from build123d import *

# Parameters (mm, degrees)
SKETCH021_W   = 231.14
SKETCH021_H   = 231.14
SKETCH021_R   = 1.5875
SKETCH021_W_2 = 7.62
SKETCH021_H_2 = 7.62
PAD003_DEPTH  = 6.35
FILLET_R      = 1.27
FILLET001_R   = 1.27
SKETCH025_W   = 9
SKETCH025_H   = 18
POCKET_DEPTH  = 6.35
FILLET002_R   = 2


with BuildPart() as part:
    # Sketch021 → Pad003 (new body)
    with BuildSketch(Plane.XY):
        with Locations((0, -18.161)):
            Rectangle(SKETCH021_W, SKETCH021_H)
        with Locations((-111.76, -129.921)):
            Circle(SKETCH021_R, mode=Mode.SUBTRACT)
        with Locations((111.76, -129.921)):
            Circle(SKETCH021_R, mode=Mode.SUBTRACT)
        with Locations((111.76, 93.599)):
            Circle(SKETCH021_R, mode=Mode.SUBTRACT)
        with Locations((-111.76, 93.599)):
            Circle(SKETCH021_R, mode=Mode.SUBTRACT)
        with Locations((-76.2, 58.42)):
            Circle(SKETCH021_R, mode=Mode.SUBTRACT)
        with Locations((76.2, 58.42)):
            Circle(SKETCH021_R, mode=Mode.SUBTRACT)
        with Locations((76.2, -93.98)):
            Circle(SKETCH021_R, mode=Mode.SUBTRACT)
        with Locations((-76.2, -93.98)):
            Circle(SKETCH021_R, mode=Mode.SUBTRACT)
        with BuildLine():
            Line((-86.995, 74.968261), (-86.995, 78.994))
            ThreePointArc((-86.995, 78.994), (-90.17, 82.169), (-93.345, 78.994))
            Line((-93.345, 78.994), (-93.345, 74.968261))
            ThreePointArc((-93.345, 74.968261), (-90.17, 63.119), (-86.995, 74.968261))
        make_face(mode=Mode.SUBTRACT)
        with Locations((7.62, 86.36)):
            Rectangle(SKETCH021_W_2, SKETCH021_H_2, mode=Mode.SUBTRACT)
        with Locations((-22.86, 86.36)):
            Rectangle(SKETCH021_W_2, SKETCH021_H_2, mode=Mode.SUBTRACT)
        with Locations((-38.1, 86.36)):
            Rectangle(SKETCH021_W_2, SKETCH021_H_2, mode=Mode.SUBTRACT)
        with Locations((-7.62, 86.36)):
            Rectangle(SKETCH021_W_2, SKETCH021_H_2, mode=Mode.SUBTRACT)
        with Locations((-68.58, 86.36)):
            Rectangle(SKETCH021_W_2, SKETCH021_H_2, mode=Mode.SUBTRACT)
        with Locations((-53.34, 86.36)):
            Rectangle(SKETCH021_W_2, SKETCH021_H_2, mode=Mode.SUBTRACT)
        with BuildLine():
            Line((86.995, 78.994), (86.995, 74.968261))
            ThreePointArc((86.995, 74.968261), (90.17, 63.119), (93.345, 74.968261))
            Line((93.345, 78.994), (93.345, 74.968261))
            ThreePointArc((93.345, 78.994), (90.17, 82.169), (86.995, 78.994))
        make_face(mode=Mode.SUBTRACT)
        with BuildLine():
            Line((-86.995, -111.290261), (-86.995, -115.316))
            ThreePointArc((-93.345, -115.316), (-90.17, -118.491), (-86.995, -115.316))
            Line((-93.345, -115.316), (-93.345, -111.290261))
            ThreePointArc((-86.995, -111.290261), (-90.17, -99.441), (-93.345, -111.290261))
        make_face(mode=Mode.SUBTRACT)
        with BuildLine():
            Line((93.345, -111.290261), (93.345, -115.316))
            ThreePointArc((86.995, -115.316), (90.17, -118.491), (93.345, -115.316))
            Line((86.995, -115.316), (86.995, -111.290261))
            ThreePointArc((93.345, -111.290261), (90.17, -99.441), (86.995, -111.290261))
        make_face(mode=Mode.SUBTRACT)
    extrude(amount=-PAD003_DEPTH)

    # Fillet
    fillet_edges = [part.edges().sort_by_distance(p)[0] for p in [
        (-72.39, 90.17, -3.175),
        (-64.77, 90.17, -3.175),
        (-64.77, 82.55, -3.175),
        (-72.39, 82.55, -3.175),
        (-57.15, 90.17, -3.175),
        (-49.53, 90.17, -3.175),
        (-49.53, 82.55, -3.175),
        (-57.15, 82.55, -3.175),
        (-41.91, 90.17, -3.175),
        (-34.29, 90.17, -3.175),
        (-34.29, 82.55, -3.175),
        (-41.91, 82.55, -3.175),
        (-26.67, 90.17, -3.175),
        (-19.05, 90.17, -3.175),
        (-19.05, 82.55, -3.175),
        (-26.67, 82.55, -3.175),
        (-11.43, 90.17, -3.175),
        (-3.81, 90.17, -3.175),
        (-3.81, 82.55, -3.175),
        (-11.43, 82.55, -3.175),
        (3.81, 90.17, -3.175),
        (11.43, 90.17, -3.175),
        (11.43, 82.55, -3.175),
        (3.81, 82.55, -3.175),
    ]]
    fillet(fillet_edges, radius=FILLET_R)

    # Fillet001
    fillet001_edges = [part.edges().sort_by_distance(p)[0] for p in [
        (-93.345, 74.968261, -3.175),
        (-86.995, 74.968261, -3.175),
        (93.345, 74.968261, -3.175),
        (86.995, 74.968261, -3.175),
        (93.345, -111.290261, -3.175),
        (86.995, -111.290261, -3.175),
        (-93.345, -111.290261, -3.175),
        (-86.995, -111.290261, -3.175),
    ]]
    fillet(fillet001_edges, radius=FILLET001_R)

    # Sketch025 (on Face86 of Fillet001) → Pocket (cut)
    with BuildSketch(Plane(origin=(0, 0, -6.35), x_dir=(1, 0, 0), z_dir=(0, 0, -1))):
        with Locations((60.5, -64.409)):
            Rectangle(SKETCH025_W, SKETCH025_H)
    pocket = extrude(amount=-POCKET_DEPTH, mode=Mode.SUBTRACT)

    # Mirrored: Pocket across YZ
    add(pocket.mirror(Plane.YZ), mode=Mode.SUBTRACT)

    # Fillet002
    fillet002_edges = [part.edges().sort_by_distance(p)[0] for p in [
        (-65, 73.409, -3.175),
        (-56, 73.409, -3.175),
        (-56, 55.409, -3.175),
        (-65, 55.409, -3.175),
        (56, 73.409, -3.175),
        (65, 73.409, -3.175),
        (65, 55.409, -3.175),
        (56, 55.409, -3.175),
    ]]
    fillet(fillet002_edges, radius=FILLET002_R)


with BuildPart() as part_1:
    # Body030 placement: moved
    add(part.part.moved(Location((0, 0, -2.54))))


solid = part_1.part
The listing builds one solid part. Answer for the finished solid, in the listing's coordinates (mm). Round coordinates to 2 decimals unless told otherwise and drop trailing zeros. Order: outer loops, then holes, each group sorted by start corner. A loop starts at its lowest first (then second) coordinate and runs counter-clockwise, first axis right, second up. Notation, with made-up numbers: M 36.25,52.5 L 52.25,52.5 A21 ccw 52.25,69.5 Z; hole C 28.5,22 d7. An arc over 180 degrees is marked long. Answer in a Markdown table with one row per item. Add a question column.
1) Determine the mould class of faces 1 (the face through (-11.43, 86, -6)), 2 (the face through (-2, -133.731, -6)) for opening direction Y: pulls with the +Y half, pulls with the -Y half, needs draft (parallel to the pull), parting line crosses it, or undercut.
2) The part is cut by section B-B on z = -4. Count the separate pieces of the cut face and the enclosed holes in it, plus the area to 3 significant figures.
3) The part is cut by section A-A on x = -90.17. Determine the outline of the cut face in (y, z), plus the area to 3 significant figures.
4) A flat-ended cylindrical pin translates along its axis: pin 1 Ø5 at (x, y) = (111.76, 93.599) entering from +Z. Find the tip coordinate at first contact, or state that the pin passes through.
5) Consider line 1 along Y through (x, z) = (-76.2, -6.5); line 2 along X through (y, z) = (-93.98, -5.25); line 3 along Y through (x, z) = (111.76, -6.5). Determine where each line is inside the solid, lowest interval first. Write a range as from..to.
Findings below:
| question | item | result |
|---|---|---|
| 1 | face 1 | undercut |
| 1 | face 2 | pulls with the -Y half |
| 2 | separate pieces | 1 |
| 2 | enclosed holes | 20 |
| 2 | area | 52,000 mm² |
| 3 | outline | M -133.73,-8.89 L -118.49,-8.89 L -118.49,-2.54 L -133.73,-2.54 Z; M -99.44,-8.89 L 63.12,-8.89 L 63.12,-2.54 L -99.44,-2.54 Z; M 82.17,-8.89 L 97.41,-8.89 L 97.41,-2.54 L 82.17,-2.54 Z |
| 3 | area | 1,230 mm² |
| 4 | pin 1 | stops at z = -2.54 |
| 5 | line 1 | y = -133.73..-95.57, -92.39..56.83, 60.01..97.41 |
| 5 | line 2 | x = -115.57..-77.79, -74.61..74.61, 77.79..115.57 |
| 5 | line 3 | y = -133.73..-131.51, -128.33..92.01, 95.19..97.41 |
